from build123d import *

# Parameters (mm, degrees)
CROQUIS1_R              = 1.7
SALIENTE_EXTRUIR1_DEPTH = 12
CROQUIS2_R              = 1.7
TORNILLO_DEPTH          = 10
TUERCA_DEPTH            = 4


with BuildPart() as part:
    # Croquis1 → Saliente-Extruir1 (new body, symmetric)
    with BuildSketch(Plane.XY):
        with BuildLine():
            Line((-4, -3), (-4, -28))
            Line((-4, -28), (4, -28))
            Line((4, -28), (4, -3))
            ThreePointArc((4, -3), (0, 5), (-4, -3))
        make_face()
        Circle(CROQUIS1_R, mode=Mode.SUBTRACT)
        with BuildLine():
            Line((1.6, -8), (1.6, -16))
            ThreePointArc((1.6, -16), (0, -17.6), (-1.6, -16))
            Line((-1.6, -16), (-1.6, -8))
            ThreePointArc((-1.6, -8), (0, -6.4), (1.6, -8))
        make_face(mode=Mode.SUBTRACT)
    extrude(amount=SALIENTE_EXTRUIR1_DEPTH, both=True)

    # Croquis2 → TORNILLO (cut)
    with BuildSketch(Plane.XZ.offset(28)):
        with Locations((0, -7)):
            Circle(CROQUIS2_R)
    tornillo = extrude(amount=-TORNILLO_DEPTH, mode=Mode.SUBTRACT)

    # Croquis3 → TUERCA (cut)
    with BuildSketch(Plane(origin=(0, -24.2, 0), x_dir=(-1, 0, 0), z_dir=(0, -1, 0))):
        Polygon((1.703183294, 9.95), (5, 9.95), (5, 4.05), (1.703183294, 4.05), (-1.703183294, 4.05), (-3.406366588, 7), (-1.703183294, 9.95), align=None)
    tuerca = extrude(amount=-TUERCA_DEPTH, mode=Mode.SUBTRACT)

    # Simetría1: TORNILLO, TUERCA across plane
    add(tornillo.mirror(Plane.XY), mode=Mode.SUBTRACT)
    add(tuerca.mirror(Plane.XY), mode=Mode.SUBTRACT)


solid = part.part
Geometry check sheet. Reference: the model listing, model coordinates, mm. A direction names the side the tool comes from. Round coordinates to 2 decimals unless told otherwise and drop trailing zeros. Order: outer loops, then holes, each group sorted by start corner. A loop starts at its lowest first (then second) coordinate and runs counter-clockwise, first axis right, second up. Notation, with made-up numbers: M -20.75,53.25 L 9.25,53.25 A8 ccw 9.25,65.25 Z; hole C -14.5,76 d4. An arc over 180 degrees is marked long. Write each question's results on one line, items separated by ' | '. Start each with the question number.
1. Cross-section at A-A on z = -2.75. Record the boundary of the cut face in (x, y).
2. Cross-section at C-C on y = -17. Record the boundary of the cut face in (x, z), plus the area to 3 significant figures.
3. Cross-section at B-B on x = -3. Record the boundary of the cut face in (y, z), plus the area to 3 significant figures.
4. Go/stop test with flat-tipped pins: P1, Ø1, axis at y = -24.5, z = -8.5, coming from the -X side; P2, Ø4, axis at x = 3, z = -7.5, coming from the +Y side; P3, Ø1, axis at x = -4, z = -9, coming from the +Y side. Record where each tip stops, or that it passes through.
5. Cross-section at D-D on z = 6.25. Record the boundary of the cut face in (x, y).
6. Material ranges on L1, parallel to Z at x = 0, y = -19.4; L2, parallel to Z at x = -0.5, y = -21; L3, parallel to X at y = -13.5, z = 9.75, recorded low to high. Write a range as from..to.
7. Draft check along X on faces 1 (the face through (2.54, -22.23, 5.5)), 2 (the face through (-2, -20.2, -7)), 3 (the face through (-0.37, -19.12, 8.66)). Enter one of: pulls with the +X half, pulls with the -X half, needs draft (parallel to the pull), parting line crosses it, or undercut.
8. Set-up check for faces 4 (the face through (0, -18, -7)), 5 (the face through (-1, -22, 9.95)), 6 (the face through (-2, -11, -12)), 7 (the face through (0, -28, 0)), 8 (the face through (1.6, -12, 0)): record each of +Z, -Z, +X, -X, +Y, -Y from which the full face is reachable in a straight line by a thin tool's end or side.
Resolved:
1) outline: M -4,-28 L 4,-28 L 4,-3 A5 ccw long -4,-3 Z; hole C 0,0 d3.4; hole M -1.6,-16 A1.6 ccw 1.6,-16 L 1.6,-8 A1.6 ccw -1.6,-8 Z
2) outline: M -4,-12 L -1.25,-12 L -1.25,12 L -4,12 Z; M 1.25,-12 L 4,-12 L 4,12 L 1.25,12 Z | area: 132 mm2
3) outline: M -28,-12 L 4,-12 L 4,12 L -28,12 Z; hole M -24.2,-9.95 L -20.2,-9.95 L -20.2,-4.05 L -24.2,-4.05 Z; hole M -24.2,4.05 L -20.2,4.05 L -20.2,9.95 L -24.2,9.95 Z | area: 721 mm2
4) P1: x = -4 | P2: y = 4.9 | P3: y = 3.57
5) outline: M -4,-28 L -1.53,-28 L -1.53,-24.2 L -4,-24.2 Z; M -4,-20.2 L -1.53,-20.2 L -1.53,-18 L 1.53,-18 L 1.53,-20.2 L 2.97,-20.2 L 2.97,-24.2 L 1.53,-24.2 L 1.53,-28 L 4,-28 L 4,-3 A5 ccw long -4,-3 Z; hole C 0,0 d3.4; hole M -1.6,-16 A1.6 ccw 1.6,-16 L 1.6,-8 A1.6 ccw -1.6,-8 Z
6) L1: -12..-8.7, -5.3..5.3, 8.7..12 | L2: -12..-9.95, -4.05..4.05, 9.95..12 | L3: -4..-1.6, 1.6..4
7) face 1: pulls with the -X half | face 2: needs draft | face 3: undercut
8) face 4: -Y | face 5: -X | face 6: -Z, +X, -X, +Y, -Y | face 7: +Z, -Z, +X, -X, -Y | face 8: +Z, -Z
